Geometry check sheet. Reference: the model listing, model coordinates, mm. Face numbers are marked on the shaded views. A direction names the side the tool comes from. Give positions to 0.01 mm unless a question says otherwise; leave off trailing zeros. Write each loop counter-clockwise with the first axis right and the second up, starting at its lowest first coordinate (ties: lowest second). Pieces come first, ordered by that corner, then holes. Notation, with made-up numbers: (45.5, 81.25) -> (83.5, 81.25) arc R26 ccw to (83.5, 99.25) -> close; hole circle Ø1 at (-39, 64.25). An arc over 180 degrees is marked (long way). One line per item, written item: value.
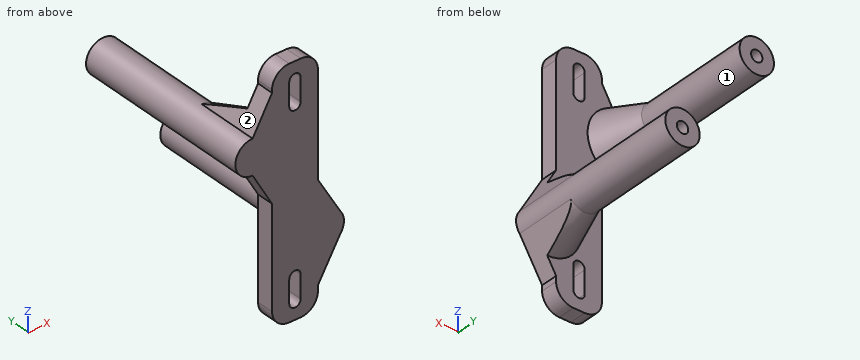
Autodesk Inventor part; units mm, degrees
ref_plane "YZ Plane" through (0, 0, 0) normal (1, 0, 0) x (0, 1, 0)
ref_plane "XZ Plane" through (0, 0, 0) normal (0, 1, 0) x (-1, 0, 0)
ref_plane "XY Plane" through (0, 0, 0) normal (0, 0, 1) x (1, 0, 0)
sketch "Sketch1" plane through (0, 0, 0) normal (0, 1, 0) x (-1, 0, 0)
  arc A0 (-1, 14) -> (1, 14) centre (0, 14) ccw
  line L0 (0, -43.0187) -> (0, 32.3947)
  arc A1 (1, 18) -> (-1, 18) centre (0, 18) ccw
  line L1 (1, 18) -> (1, 14)
  line L2 (-1, 14) -> (-1, 18)
  line L3 (0, 18) -> (0, 16)
  line L4 (3.8037, 16) -> (0, 16) construction
  line L5 (14.482, 0) -> (-14.022, 0) construction
  arc A2 (1, -14) -> (-1, -14) centre (0, -14) ccw
  arc A3 (-1, -18) -> (1, -18) centre (0, -18) ccw
  line L6 (1, -18) -> (1, -14)
  line L7 (-1, -14) -> (-1, -18)
  line L8 (3.8037, -16) -> (0, -16) construction
  line L9 (1, 21) -> (-1, 21)
  line L10 (-4, 18) -> (-4, -18)
  line L11 (-1, -21) -> (1, -21)
  line L12 (4, -18) -> (4, 18)
  arc A4 (4, 18) -> (1, 21) centre (1, 18) ccw
  arc A5 (-1, 21) -> (-4, 18) centre (-1, 18) ccw
  arc A6 (-4, -18) -> (-1, -21) centre (-1, -18) ccw
  arc A7 (1, -21) -> (4, -18) centre (1, -18) ccw
  line L13 (9.95, -10.51) -> (-9.95, -10.51) construction
  line L14 (-9.95, -10.51) -> (-9.95, 10.51) construction
  line L15 (9.95, 10.51) -> (9.95, -10.51) construction
  circle A8 centre (7.41, 8.51) radius 1
  circle A9 centre (-5.55, -8.49) radius 0.75 construction
  line L16 (0, -32.2454) -> (0, -10.51) construction
  line L17 (9.95, 0) -> (-9.95, 0) construction
  line L18 (9.95, 10.51) -> (-9.95, 10.51) construction
  line L19 (4, 10.51) -> (9, 10.51) construction
  line L20 (9, 10.51) -> (9, 6.51) construction
  line L21 (9, 6.51) -> (4, 6.51) construction
  line L22 (4, 6.51) -> (4, 10.51)
  line L23 (7.41, 8.51) -> (9.1387, 8.51) construction
  circle A10 centre (7.41, 8.51) radius 3
  line L24 (7.41, 11.51) -> (4, 11.51)
  line L25 (7.41, 5.51) -> (4, 5.51)
  arc A11 (-4, -7.2261) -> (-4, -9.7539) centre (-5.55, -8.49) ccw construction
  line L26 (-5.55, -6.49) -> (-4, -6.49) construction
  line L27 (-5.55, -10.49) -> (-4, -10.49) construction
  circle A12 centre (-5.55, -8.49) radius 2 construction
  line L28 (-7.55, -8.49) -> (-7.55, -26.4012) construction
  circle A13 centre (-5.55, -8.49) radius 3
  circle A14 centre (-5.55, -8.49) radius 1
  point P0 (0, 0)
  point P1 (0, 21)
  point P2 (0, 19)
  point P3 (-5.55, -6.94)
  point P4 (-4, -6.94)
  point P5 (-5.55, -10.04)
  point P6 (-4, -10.04)
  point P7 (4, 5.51)
  point P8 (4, 11.51)
  point P9 (-4, -9.7539)
  point P10 (-4, -9.7539)
  dimension "d4" = 2
  dimension "d7" = 2
  dimension "d14" = 2
  dimension "d15" = 16
  dimension "d16" = 2
  dimension "d17" = 2
  dimension "d18" = 16
  dimension "d19" = 42
  dimension "d21" = 8
  dimension "d22" = 3
  dimension "d24" = 19.9
  dimension "d31" = 2.54
  dimension "d33" = 17
  dimension "d34" = 19.9
  dimension "d36" = 15.5
  dimension "d37" = 5
  dimension "d38" = 4
  dimension "d39" = 2
  dimension "d40" = 1.5
  dimension "d45" = 4
  dimension "d46" = 6
  dimension "d51" = 7.55
  dimension "d64" = 6
  dimension "d65" = 2
extrude "Extrusion2" add sketch "Sketch1" along normal blind 32 contours A10 | A8
extrude "Extrusion3" add sketch "Sketch1" along normal blind 32 contours A13 L10 | L10 A13 | A14
extrude "Extrusion4" add sketch "Sketch1" along normal blind 3 contours A0 L0 A2 L7 A3 L11 A6 L10 A13 A5 L9 A1 L2 | A0 L1 A1 L0 L9 A4 L12 A7 L11 A3 L6 A2 | L24 A10 L25 L12 | A13 L10 picked at (-3.0537, -8.3357)
chamfer "Chamfer1" distance 4 distance2 6 2 edges at (4, 1.5, -11.0586) (4, 1.5, -5.9214) measured on face at (8.55, 10.6667, -8.49)
chamfer_without_effect "Chamfer2"
chamfer "Chamfer3" distance 6 distance2 3.4 1 edges at (-4, 1.5, 5.51) measured on face at (-4, 1, -10.1633)
chamfer "Chamfer4" distance 3.4 distance2 6 1 edges at (-4, 1.5, 11.51) measured on face at (-6.2733, 1, 11.51)
chamfer "Chamfer5" distance 8 angle 20 1 edges at (-4.41, 3, 8.51)
chamfer "Chamfer6" distance 8 angle 20 2 edges at (4.586, 3, -5.6491) (4.586, 3, -11.3309) measured on face at (8.3281, 21.3333, -9.6224)
sketch "Sketch2" plane through (-7.41, 32, 8.51) normal (0, 1, 0) x (1, 0, 0)
  circle A0 centre (0, 0) radius 3
  circle A1 centre (0, 0) radius 1
  circle A2 centre (12.96, 17) radius 3
  circle A3 centre (12.96, 17) radius 1
  point P0 (7.41, 8.51)
  dimension "d72" = 2
  dimension "d73" = 2
extrude "Extrusion5" cut sketch "Sketch2" against normal blind 8 contours A1 | A3
properties part number "supporto_mb1202"
1) Sectioned sample at C-C on y = 16. Record the cut outline in (x, z).
Verdict:
outline: circle Ø6 at (-7.41, 8.51); circle Ø6 at (5.55, -8.49)
2) Sectioned sample at D-D on z = -1.5. Record the cut outline in (x, y).
Verdict:
outline: (-4, 0) -> (4.92, 0) -> (4.92, 3) -> (-4, 3) -> close
3) Depth check by flat-ended pin: pin 1 Ø0.9 at (y, z) = (2, 15.5) entering from +X; pin 2 Ø2 at (y, z) = (9.5, -12.5) entering from +X; pin 3 Ø2.5 at (y, z) = (1, 15) entering from -X. Enter the tip coordinate at first touch or a pass-through.
Verdict:
pin 1: x = 4
pin 2: x = 7.24
pin 3: x = -6.13
4) Tool access check on the marked faces 1 and 2. Record the directions out of +Z, -Z, +X, -X, +Y, -Y that give a thin tool (end or side, any length) a straight path to the whole face; none if there is none.
Verdict:
face 1: +Y
face 2: +Z, -X, +Y, -Y
5) Scan lines: probe 1 along X at (y, z) = (27.25, 8.51); probe 2 along Z at (x, y) = (-7.41, 28.5); probe 3 along X at (y, z) = (26.25, -8.49). Record each from-to range of solid material in increasing order.
Verdict:
probe 1: -10.41 to -8.41, -6.41 to -4.41
probe 2: 5.51 to 7.51, 9.51 to 11.51
probe 3: 2.55 to 4.55, 6.55 to 8.55
6) Sectioned sample at A-A on z = 8.51. Record the cut outline in (x, y), plus the area to 3 significant figures.
Verdict:
outline: (-10.41, 0) -> (4, 0) -> (4, 3) -> (-1.5, 3) -> (-4.41, 11) -> (-4.41, 32) -> (-6.41, 32) -> (-6.41, 24) -> (-8.41, 24) -> (-8.41, 32) -> (-10.41, 32) -> close
area: 213 mm^2
